CAD build for the part. Positions are in the model's coordinates, mm. A direction names the side the tool comes from. Round coordinates to 2 decimals unless told otherwise and drop trailing zeros. Loops run counter-clockwise (first coordinate to the right, second up) from the corner with the lowest first, then second, coordinate; pieces in that order, holes last.
```python
from build123d import *

# Parameters (mm, degrees)
CROQUIS1_R              = 400
SALIENTE_EXTRUIR1_DEPTH = 520
CROQUIS3_R              = 50
CROQUIS2_R              = 400
CROQUIS4_W              = 100
CROQUIS4_H              = 100
SALIENTE_EXTRUIR2_DEPTH = 50


with BuildPart() as part:
    # Croquis1 → Saliente-Extruir1 (new body)
    with BuildSketch(Plane(origin=(0, 0, 0), x_dir=(1, 0, 0), z_dir=(0, 1, 0))):
        with Locations(Location((0, 0, 0), (0, 0, 270))):
            Circle(CROQUIS1_R)
    extrude(amount=-SALIENTE_EXTRUIR1_DEPTH)

    # Croquis3 → Recubrir1 section 0
    with BuildSketch(Plane(origin=(0, -900, 0), x_dir=(1, 0, 0), z_dir=(0, 1, 0))):
        Circle(CROQUIS3_R)
    # Croquis2 → Recubrir1 section 1
    with BuildSketch(Plane.XZ.offset(520)):
        Circle(CROQUIS2_R)
    loft()

    # Croquis4 → Saliente-Extruir2 (add)
    with BuildSketch(Plane.XZ.offset(900)):
        Rectangle(CROQUIS4_W, CROQUIS4_H)
    extrude(amount=SALIENTE_EXTRUIR2_DEPTH)


solid = part.part
```
Item 1: Two-plate mould, pull along Y, no slides. Class faces 5 (the flat face through (6, 0, -6)), 6 (the flat face through (-1, -950, 1)), 7 (the flat face through (-40, -900, 38)): released by +Y, released by -Y, zero draft, split by the parting line, or undercut.
Answers follow:
face 5: released by +Y
face 6: released by -Y
face 7: undercut
Item 2: Cut at A-A, the plane y = -708. Give the cut face in (x, z).
Answers follow:
outline: circle Ø453.68 at (0, 0)
Item 3: 3-axis set-ups, long thin cutter, end or side, ignore diameter. For faces 1 (the flat face through (-1, -925, -50)), 2 (the flat face through (50, -925, -1)), 3 (the flat face through (-1, -925, 50)), 4 (the flat face through (-50, -925, -1)): which of +Z, -Z, +X, -X, +Y, -Y reach the whole face in a straight line?
Answers follow:
face 1: -Z, +X, -X, -Y
face 2: +Z, -Z, +X, -Y
face 3: +Z, +X, -X, -Y
face 4: +Z, -Z, -X, -Y
Item 4: Flat gauge pins, fed straight in: P1, Ø6, axis at y = -807, z = 104, coming from the -X side; P2, Ø12, axis at y = -354, z = -132, coming from the +X side; P3, Ø5, axis at x = -84.5, y = -660, coming from the +Z side. Where does each tip first touch, or does it go through?
Answers follow:
P1: stops at x = -92.54
P2: stops at x = 379.64
P3: stops at z = 260.1
Item 5: Probe line 1 (X direction, y = -681, z = 131); line 2 (Z direction, x = 206, y = -661.5); line 3 (X direction, y = -614, z = 86). List the from-to ranges inside material, lowest first.
Answers follow:
line 1: x = -214.94 to 214.94
line 2: z = -174.03 to 174.03
line 3: x = -301.39 to 301.39
